Read the model definition and answer for the solid it produces. Units are mm, in the model's axes. A direction names the side the tool comes from. Coordinates: 2 decimals unless noted, no trailing zeros. Loops run counter-clockwise (first coordinate to the right, second up) from the corner with the lowest first, then second, coordinate; pieces in that order, holes last. Notation, with made-up numbers: (57, 24.25) - (107, 24.25) arc R8 ccw to (107, 36.25) - close; hole circle Ø2 at (60.25, -27.5). An arc over 180 degrees is marked (long way). Use one line per item in the form item = value.
from build123d import *

# Parameters (mm, degrees)
F0_R      = 3.175
F1_DEPTH  = 2
F3_DEPTH  = 88.9
F5_DEPTH  = 88.9
F6_W      = 44.45
F6_H      = 57.15
F7_DEPTH  = 25.4
F8_W      = 44.45
F8_H      = 57.15
F9_DEPTH  = 25.4
F10_R     = 4.7625
F11_DEPTH = 88.9
F12_R     = 5.08
F13_R     = 5.08


with BuildPart() as f1:
    # F0 (on Top) → F1 (new body)
    with BuildSketch(Plane.XY):
        with BuildLine():
            ThreePointArc((6.35, 12.7), (0, 6.35), (6.35, 0))
            Line((6.35, 0), (31.75, 0))
            Line((31.75, 0), (31.75, 25.4))
            Line((31.75, 25.4), (63.5, 25.4))
            Line((63.5, 25.4), (63.5, 41.275))
            Line((63.5, 41.275), (31.75, 41.275))
            Line((31.75, 41.275), (31.75, 98.425))
            Line((31.75, 98.425), (63.5, 98.425))
            Line((63.5, 98.425), (63.5, 114.3))
            Line((63.5, 114.3), (31.75, 114.3))
            Line((31.75, 114.3), (31.75, 139.7))
            Line((31.75, 139.7), (6.35, 139.7))
            ThreePointArc((6.35, 139.7), (0, 133.35), (6.35, 127))
            Line((6.35, 127), (19.05, 127))
            Line((19.05, 127), (19.05, 12.7))
            Line((19.05, 12.7), (6.35, 12.7))
        make_face()
        with Locations((6.35, 6.35)):
            Circle(F0_R, mode=Mode.SUBTRACT)
        with Locations((6.35, 133.35)):
            Circle(F0_R, mode=Mode.SUBTRACT)
    extrude(amount=F1_DEPTH)

    # F2 (on face) → F3 (join, through all)
    with BuildSketch(Plane.XZ.offset(-25.4)):
        with BuildLine():
            ThreePointArc((56.5092743605, 9.7027625733), (55.1601848792, 11.7076454488), (55.0783732507, 9.2925047427))
            ThreePointArc((55.0783732507, 9.2925047427), (60.2557743605, 1), (65.4331754703, 9.2925047427))
            ThreePointArc((65.4331754703, 9.2925047427), (65.3513638418, 11.7076454488), (64.0022743605, 9.7027625733))
            ThreePointArc((64.0022743605, 9.7027625733), (60.2557743605, 2), (56.5092743605, 9.7027625733))
        make_face()
        with BuildLine():
            ThreePointArc((46.1272743605, 9.7027625733), (42.3807743605, 2), (38.6342743605, 9.7027625733))
            ThreePointArc((38.6342743605, 9.7027625733), (37.2851848792, 11.7076454488), (37.2033732507, 9.2925047427))
            ThreePointArc((37.2033732507, 9.2925047427), (42.3807743605, 1), (47.5581754703, 9.2925047427))
            ThreePointArc((47.5581754703, 9.2925047427), (47.4763638418, 11.7076454488), (46.1272743605, 9.7027625733))
        make_face()
    extrude(amount=-F3_DEPTH)

    # F4 (on face) → F5 (join, through all)
    with BuildSketch(Plane.XZ.offset(-25.4)):
        Polygon((63.5, 0), (65.4964292905, 4.3662650043), (63.5, 2), align=None)
    extrude(amount=-F5_DEPTH)

    # F6 (on face) → F7 (cut)
    with BuildSketch(Plane(origin=(0, 0, 0), x_dir=(1, 0, 0), z_dir=(0, 0, -1))):
        with Locations((53.975, -69.85)):
            Rectangle(F6_W, F6_H)
    extrude(amount=-F7_DEPTH, mode=Mode.SUBTRACT)

    # F8 (on face) → F9 (cut)
    with BuildSketch(Plane.XY.offset(2)):
        with Locations((41.275, 69.85)):
            Rectangle(F8_W, F8_H)
    extrude(amount=F9_DEPTH, mode=Mode.SUBTRACT)

    # F10 (on face) → F11 (cut, through all)
    with BuildSketch(Plane.XZ.offset(-25.4)):
        with Locations((42.3807743605, 6.7625)):
            Circle(F10_R)
        with Locations((60.2557743605, 6.7625)):
            Circle(F10_R)
    extrude(amount=-F11_DEPTH, mode=Mode.SUBTRACT)

    # F12
    f12_edges = [f1.edges().sort_by_distance(p)[0] for p in [
        (31.75, 0, 1),
        (31.75, 25.4, 1),
        (31.75, 41.275, 1),
        (31.75, 98.425, 1),
        (31.75, 114.3, 1),
        (31.75, 139.7, 1),
        (19.05, 127, 1),
        (19.05, 12.7, 1),
    ]]
    fillet(f12_edges, radius=F12_R)

    # F13
    f13_edges = [f1.edges().sort_by_distance(p)[0] for p in [
        (63.5, 33.3375, 0),
        (63.5, 106.3625, 0),
    ]]
    fillet(f13_edges, radius=F13_R)


solid = f1.part
Item 1: The part is cut by section A-A on y = 6.35. Give the vertices of the cut face in (x, z) (3 decimals).
Results below:
outline = (0, 0) - (3.175, 0) - (3.175, 2) - (0, 2) - close; (9.525, 0) - (31.75, 0) - (31.75, 2) - (9.525, 2) - close
Item 2: Which of the six approach directions +Z, -Z, +X, -X, +Y, -Y give full straight-line access (tool end or side, diameter ignored) to faces 1 (the flat face through (50.1, 114.3, 1.6)), 2 (the flat face through (50, 41.275, 1)), 3 (the cylindrical face through (4.01, 8.496, 0.986)), 4 (the cylindrical face through (17.522, 125.551, 1.014))?
Results below:
face_1 = +Z, -Z, +X, +Y
face_2 = +Z, -Z, +X
face_3 = +Z, -Z
face_4 = +Z, -Z, -X
Item 3: Find the intervals of material crossed by L1, parallel to X at y = 133, z = 0.5; L2, parallel to X at y = 35, z = 2.5; L3, parallel to Y at x = 6.35, z = 1.45 (3 decimals), in increasing order.
Results below:
L1 = 0.01 to 3.19, 9.51 to 31.75
L2 = 38.5 to 40.26, 44.51 to 46.26, 56.38 to 58.13, 62.38 to 64.61
L3 = 0 to 3.175, 9.525 to 12.7, 127 to 130.175, 136.525 to 139.7
Item 4: The part is cut by section C-C on y = 23.5. Give the vertices of the cut face in (x, z).
Results below:
outline = (19.05, 0) - (32.87, 0) - (32.87, 2) - (19.05, 2) - close
Item 5: The part is cut by section D-D on y = 95. Give the vertices of the cut face in (x, z).
Results below:
outline = (19.05, 0) - (32.03, 0) - (32.03, 2) - (19.05, 2) - close
Item 6: For a pull along Z with two mould halves and no side action, classify faces 5 (the cylindrical face through (62.948, 106.474, 0.784)), 6 (the cylindrical face through (30.301, 1.528, 1.014)), 7 (the cylindrical face through (65.394, 106.251, 11.695)) as +Z half, -Z half, draft (parallel to the pull), parting line (faces both ways), or undercut.
Results below:
face_5 = -Z half
face_6 = draft
face_7 = undercut
Item 7: The part is cut by section B-B on z = 7.25. Count the separate pieces of the cut face and the enclosed holes in it, plus the area to 3 significant figures.
Results below:
separate_pieces = 8
enclosed_holes = 0
area = 128 mm²
Item 8: Each of these flat-tipped pins is pushed along its axis until it touches: P1, Ø10, axis at x = 6.35, y = 6.35, coming from the +Z side; P2, Ø0.6, axis at y = 127.5, z = 1, coming from the +X side; P3, Ø5, axis at y = 36.5, z = 7, coming from the -X side. Where does it stop, or does it pass through?
Results below:
P1 = 2
P2 = 31.75
P3 = 36.62
